from build123d import *

# Parameters (mm, degrees)
F1_DEPTH = 31.75


with BuildPart() as f1:
    # F0 (on Top) → F1 (new body)
    with BuildSketch(Plane.XY):
        with BuildLine():
            Line((-736.6, 0), (-25.4, 0))
            ThreePointArc((-25.4, 0), (-7.439488, 7.439488), (0, 25.4))
            Line((0, 25.4), (0, 622.3))
            Line((0, 622.3), (762, 622.3))
            Line((762, 622.3), (762, 673.1))
            Line((762, 673.1), (-762, 673.1))
            Line((-762, 673.1), (-762, 25.4))
            ThreePointArc((-762, 25.4), (-754.560512, 7.439488), (-736.6, 0))
        make_face()
    extrude(amount=F1_DEPTH)


solid = f1.part
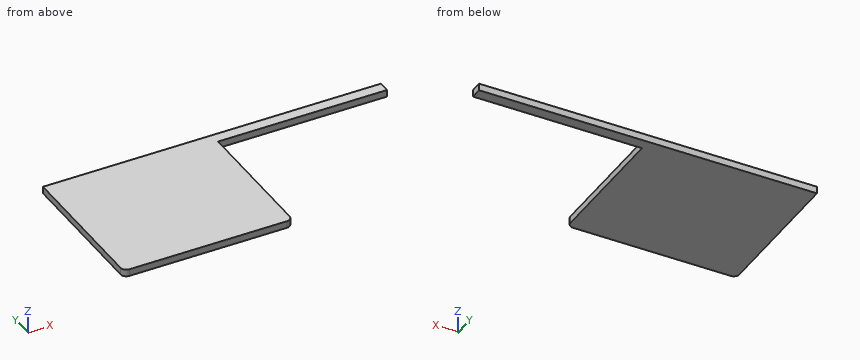
Source: CAD feature listing. Evaluate the final solid. Frame: model axes, mm. Coordinates: 2 decimals unless noted, no trailing zeros. Order: outer loops, then holes, each group sorted by start corner. A loop starts at its lowest first (then second) coordinate and runs counter-clockwise, first axis right, second up.
Item 1: First-contact query: P1, Ø12, axis at x = 15, z = 6.5, coming from the -Y side; P2, Ø4, axis at y = 393.5, z = 19, coming from the +X side. Flat tips, straight axial feed; report the tip coordinate or a pass-through.
Output values:
P1: stops at y = 622.3
P2: stops at x = 0
Item 2: Material intervals for line 1 (Y direction, x = 528, z = 10.5); line 2 (X direction, y = 255.5, z = 29.5), sorted ascending.
Output values:
line 1: y = 622.3 to 673.1
line 2: x = -762 to 0
Item 3: Cut plane C-C (x = 19). Return loops of the section in (y, z).
Output values:
outline: (622.3, 0) - (673.1, 0) - (673.1, 31.75) - (622.3, 31.75) - close
Item 4: Cut plane A-A (z = 5.5). Return loops of the section in (x, y), plus the area to 3 significant figures.
Output values:
outline: (-762, 25.4) arc R25.4 ccw to (-736.6, 0) - (-25.4, 0) arc R25.4 ccw to (0, 25.4) - (0, 622.3) - (762, 622.3) - (762, 673.1) - (-762, 673.1) - close
area: 551,000 mm2
Item 5: Cut plane B-B (y = 268). Return loops of the section in (x, z), plus the area to 3 significant figures.
Output values:
outline: (-762, 0) - (0, 0) - (0, 31.75) - (-762, 31.75) - close
area: 24,200 mm2
